Geometry check sheet. Reference: the model listing, model coordinates, mm. A direction names the side the tool comes from. Round coordinates to 2 decimals unless told otherwise and drop trailing zeros. Order: outer loops, then holes, each group sorted by start corner. A loop starts at its lowest first (then second) coordinate and runs counter-clockwise, first axis right, second up.
(1) Material ranges on line 1 along Y through (x, z) = (6, -0.75); line 2 along Z through (x, y) = (0.6, -36.8); line 3 along X through (y, z) = (-25, 3), recorded low to high.
(2) Set-up check for faces 1 (the face through (2, -28, 4)), 2 (the face through (0.986, -38.565, 4.556)): record each of +Z, -Z, +X, -X, +Y, -Y from which the full face is reachable in a straight line by a thin tool's end or side.
(3) Release check for a two-part mould opening along Z. For faces 3 (the face through (9.699, -0.285, -0.986)), 4 (the face through (0.986, -4.559, 5.834)), 5 (the face through (0.986, -57.299, 7.715)), 6 (the face through (5, -28, -2)) record: +Z half, -Z half, draft (parallel to the pull), parting line (faces both ways), or undercut.
(4) Sectioned sample at D-D (y = -51.5). Record the boundary of the cut face in (x, z), plus the area to 3 significant figures.
(5) Sectioned sample at A-A (y = -36.8). Record the boundary of the cut face in (x, z).
(6) Go/stop test with flat-tipped pins: pin 1 (4 mm diameter, centred on y = -22.5, z = 6, fed in from +X); pin 2 (4.5 mm diameter, centred on x = 6, y = -4.8, fed in from +Z); pin 3 (3.5 mm diameter, centred on x = 6, y = -36.8, fed in from +Z). Record where each tip stops, or that it passes through.
(7) Sectioned sample at C-C (x = 7). Record the boundary of the cut face in (y, z), plus the area to 3 significant figures.
(8) Sectioned sample at B-B (z = 3). Record the boundary of the cut face in (x, y), plus the area to 3 significant figures.
from build123d import *

# Parameters (mm, degrees)
F1_DEPTH = 57.6
F2_R     = 1
F3_R     = 1
F4_R     = 1
F5_R     = 1
F7_D     = 3.7
F9_D     = 3.7


with BuildPart() as f1:
    # F0 (on Front) → F1 (new body)
    with BuildSketch(Plane.XZ):
        Polygon((2, 8), (0, 8), (0, -2), (10, -2), (10, 0), (2, 0), align=None)
    extrude(amount=F1_DEPTH)

    # F2
    f2_edges = [f1.edges().sort_by_distance(p)[0] for p in [
        (1, -57.6, 8),
    ]]
    fillet(f2_edges, radius=F2_R)

    # F3
    f3_edges = [f1.edges().sort_by_distance(p)[0] for p in [
        (10, -57.6, -1),
    ]]
    fillet(f3_edges, radius=F3_R)

    # F4
    f4_edges = [f1.edges().sort_by_distance(p)[0] for p in [
        (1, 0, 8),
    ]]
    fillet(f4_edges, radius=F4_R)

    # F5
    f5_edges = [f1.edges().sort_by_distance(p)[0] for p in [
        (10, 0, -1),
    ]]
    fillet(f5_edges, radius=F5_R)

    # F7 (through all)
    with Locations(Plane.XY):
        with Locations((6, -52.8), (6, -36.8), (6, -20.8), (6, -4.8)):
            Hole(F7_D / 2)

    # F9 (through all)
    with Locations(Plane.YZ.offset(2)):
        with Locations((-52.8, 4), (-36.8, 4), (-20.8, 4), (-4.8, 4)):
            Hole(F9_D / 2)


solid = f1.part
Answer below:
1. line 1: y = -57.6 to -54.65, -50.95 to -38.65, -34.95 to -22.65, -18.95 to -6.65, -2.95 to 0
1. line 2: z = -2 to 2.15, 5.85 to 8
1. line 3: x = 0 to 2
2. face 1: +Z, +X, +Y, -Y
2. face 2: +X, -X
3. face 3: draft
3. face 4: undercut
3. face 5: +Z half
3. face 6: -Z half
4. outline: (0, -2) - (4.68, -2) - (4.68, 0) - (2, 0) - (2, 2.68) - (0, 2.68) - close; (0, 5.32) - (2, 5.32) - (2, 8) - (0, 8) - close; (7.32, -2) - (10, -2) - (10, 0) - (7.32, 0) - close
4. area: 25.5 mm2
5. outline: (0, -2) - (4.15, -2) - (4.15, 0) - (2, 0) - (2, 2.15) - (0, 2.15) - close; (0, 5.85) - (2, 5.85) - (2, 8) - (0, 8) - close; (7.85, -2) - (10, -2) - (10, 0) - (7.85, 0) - close
6. pin 1: stops at x = 2
6. pin 2: stops at z = 0
6. pin 3: passes through
7. outline: (-57.6, -2) - (-54.36, -2) - (-54.36, 0) - (-57.6, 0) - close; (-51.24, -2) - (-38.36, -2) - (-38.36, 0) - (-51.24, 0) - close; (-35.24, -2) - (-22.36, -2) - (-22.36, 0) - (-35.24, 0) - close; (-19.24, -2) - (-6.36, -2) - (-6.36, 0) - (-19.24, 0) - close; (-3.24, -2) - (0, -2) - (0, 0) - (-3.24, 0) - close
7. area: 90.3 mm2
8. outline: (0, -57.6) - (2, -57.6) - (2, -54.36) - (0, -54.36) - close; (0, -51.24) - (2, -51.24) - (2, -38.36) - (0, -38.36) - close; (0, -35.24) - (2, -35.24) - (2, -22.36) - (0, -22.36) - close; (0, -19.24) - (2, -19.24) - (2, -6.36) - (0, -6.36) - close; (0, -3.24) - (2, -3.24) - (2, 0) - (0, 0) - close
8. area: 90.3 mm2
